Geometry: see drawing. Coordinates: mm, zero at the bounding-box minimum. A direction names the side the tool comes from. Round coordinates to 2 decimals unless told otherwise and drop trailing zeros. Loops run counter-clockwise (first coordinate to the right, second up) from the corner with the lowest first, then second, coordinate; pieces in that order, holes last. Notation, with made-up numbers: (38, -3) - (74, -3) arc R8 cw to (74, 10) - close; hole circle Ø8 at (86, 89). An arc over 180 degrees is marked (long way). Use CSV: the item, a comma, the result in double quotes.
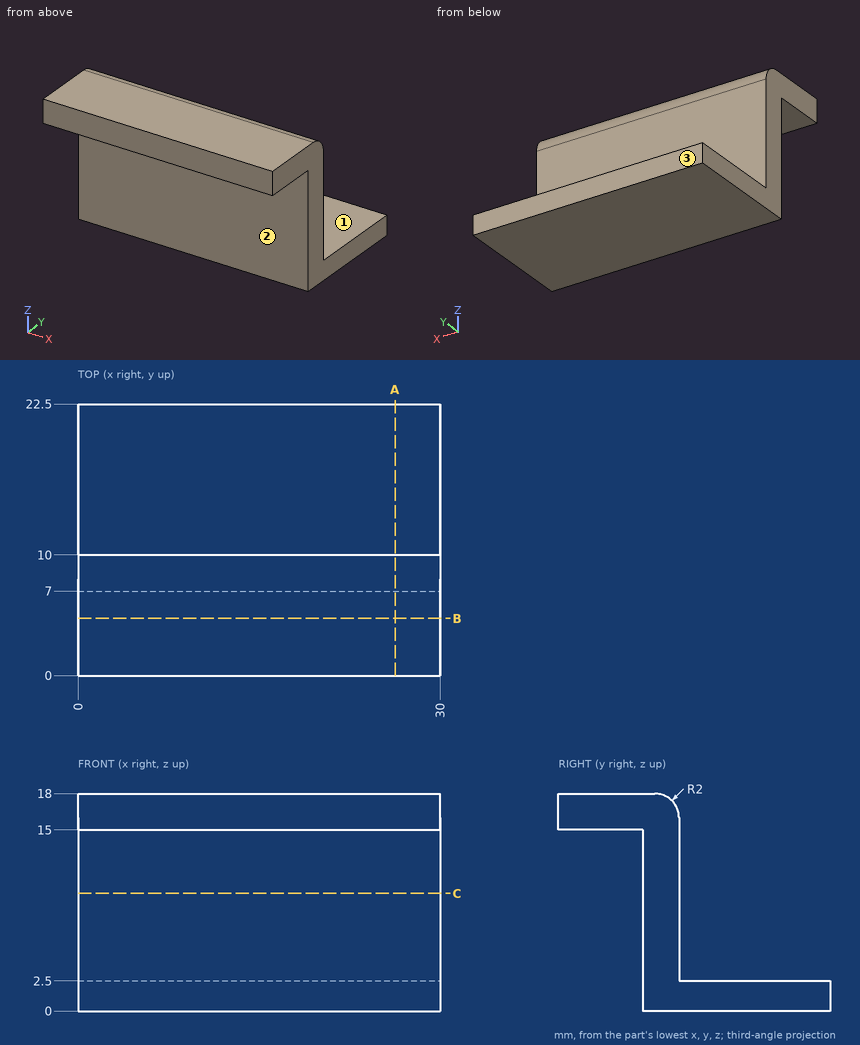
Item 1: Material intervals for line 1 (Z direction, x = 17.25, y = 19.5); line 2 (Y direction, x = 24, z = 8); line 3 (Y direction, x = 15.75, z = 16), sorted ascending.
Final values:
line 1,"z = 0 to 2.5"
line 2,"y = 7 to 10"
line 3,"y = 0 to 10"
Item 2: Pin query (flat end, axial travel): P1, Ø5.5, axis at x = 14, y = 3, coming from the -Z side; P2, Ø1, axis at x = 15, z = 9, coming from the -Y side; P3, Ø10, axis at x = 18, y = 19.5, coming from the +Z side; P4, Ø6, axis at y = 14, z = 8.5, coming from the -X side. Return the tip coordinate at first contact, or that it passes through.
Final values:
P1,"stops at z = 15"
P2,"stops at y = 7"
P3,"stops at z = 2.5"
P4,"passes through"
Item 3: Section A-A on x = 26.25. Return the cut outline in (y, z).
Final values:
outline,"(0, 15) - (7, 15) - (7, 0) - (22.5, 0) - (22.5, 2.5) - (10, 2.5) - (10, 16) arc R2 ccw to (8, 18) - (0, 18) - close"
Item 4: Reachability of the marked faces 1, 2 and 3 from +Z, -Z, +X, -X, +Y, -Y: full face, straight path, thin tool, end or side. Return the list, or none.
Final values:
face 1,"+Z, +X, -X, +Y"
face 2,"-Z, +X, -X, -Y"
face 3,"+Z, -Z, +X, -X, +Y"
Item 5: Section C-C on z = 9.75. Return the cut outline in (x, y), plus the area to 3 significant figures.
Final values:
outline,"(0, 7) - (30, 7) - (30, 10) - (0, 10) - close"
area,"90.0 mm²"
Item 6: Section B-B on y = 4.75. Return the cut outline in (x, z), plus the area to 3 significant figures.
Final values:
outline,"(0, 15) - (30, 15) - (30, 18) - (0, 18) - close"
area,"90.0 mm²"
